```python
from build123d import *

# Parameters (mm, degrees)
SKETCH1_R           = 15
BOSS_EXTRUDE1_DEPTH = 35
SKETCH3_W           = 8
SKETCH3_H           = 45
CUT_EXTRUDE1_DEPTH  = 115
SKETCH5_R           = 30
BOSS_EXTRUDE2_DEPTH = 75


with BuildPart() as part:
    # Sketch1 → Boss-Extrude1 (new body)
    with BuildSketch(Plane.XY):
        with BuildLine():
            Line((-40, 107.819293264), (-40, -107.819293264))
            ThreePointArc((-40, -107.819293264), (0, -115), (40, -107.819293264))
            Line((40, -107.819293264), (40, 107.819293264))
            ThreePointArc((40, 107.819293264), (0, 115), (-40, 107.819293264))
        make_face()
        with Locations((0, 75)):
            Circle(SKETCH1_R, mode=Mode.SUBTRACT)
        with Locations((0, -75)):
            Circle(SKETCH1_R, mode=Mode.SUBTRACT)
    extrude(amount=BOSS_EXTRUDE1_DEPTH)

    # Sketch3 → Cut-Extrude1 (cut)
    with BuildSketch(Plane(origin=(40, 0, 0), x_dir=(0, 0, -1), z_dir=(1, 0, 0))):
        with Locations((-4, 0)):
            Rectangle(SKETCH3_W, SKETCH3_H)
    extrude(amount=-CUT_EXTRUDE1_DEPTH, mode=Mode.SUBTRACT)

    # Sketch5 → Boss-Extrude2 (add)
    with BuildSketch(Plane.XY.offset(35)):
        Circle(SKETCH5_R)
    extrude(amount=BOSS_EXTRUDE2_DEPTH)


solid = part.part
```
Can you work these out from the model? Positions are in its coordinate system, mm. A direction names the side the tool comes from. Give positions to 0.01 mm unless a question says otherwise; leave off trailing zeros. Loops run counter-clockwise (first coordinate to the right, second up) from the corner with the lowest first, then second, coordinate; pieces in that order, holes last. Notation, with made-up numbers: M 37,-31.75 L 93,-31.75 A5 cw 93,-23.75 Z; hole C 46,-33.5 d4. An arc over 180 degrees is marked long. Use one line per item in the form item = value. Start each with the question number.
(1) On a 3-axis mill with a long thin cutter (end or side, diameter ignored), from which of +Z, -Z, +X, -X, +Y, -Y can I reach the whole of each face in a straight line? I mean faces 4 (the cylindrical face through (-29.97, 1.32, 71.97)), 5 (the flat face through (1, -22.5, 4)), 6 (the flat face through (40, -2, 17)). Say none if no direction works.
(2) I want a section at B-B, the plane x = 0. Write out the boundary of the cut face in (y, z).
(3) I want a section at C-C, the plane z = 22.5. Write out the boundary of the cut face in (x, y), and give its area (3 significant figures).
(4) I'm going to push flat-ended pins straight in: P1, Ø5, axis at x = -4.5, z = 64, coming from the +Y side; P2, Ø12, axis at x = 21, z = 96, coming from the -Y side; P3, Ø3, axis at x = 7, z = 90, coming from the -Y side. Where does each tip first touch, or does it pass through?
(5) Please list where these lines run through material, in increasing order: line 1 (Y direction, x = 0, z = 13.5); line 2 (Z direction, x = 19, y = 78.5); line 3 (Z direction, x = 7.5, y = -12).
(6) Thinking about a two-plate mould opening in Y: for faces 1 (the cylindrical face through (-0.6, -115, 17.3)), 2 (the flat face through (1, 22.5, 4)), 3 (the cylindrical face through (0.6, 115, 17.3)), which applies, released by +Y, released by -Y, zero draft, split by the parting line, or undercut?
(7) I want a section at A-A, the plane y = 75. Write out the boundary of the cut face in (x, z).
(8) I want a section at D-D, the plane y = 0. Write out the boundary of the cut face in (x, z).
Worked out:
q1.face_4 = +Z
q1.face_5 = -Z, +X, -X
q1.face_6 = +Z, -Z, +X, +Y, -Y
q2.outline = M -115,0 L -90,0 L -90,35 L -115,35 Z; M -60,0 L -22.5,0 L -22.5,8 L 22.5,8 L 22.5,0 L 60,0 L 60,35 L 30,35 L 30,110 L -30,110 L -30,35 L -60,35 Z; M 90,0 L 115,0 L 115,35 L 90,35 Z
q3.outline = M -40,-107.82 A115 ccw 40,-107.82 L 40,107.82 A115 ccw -40,107.82 Z; hole C 0,-75 d30; hole C 0,75 d30
q3.area = 16,600 mm²
q4.P1 = 29.93
q4.P2 = -25.98
q4.P3 = -29.49
q5.line_1 = -115 to -90, -60 to 60, 90 to 115
q5.line_2 = 0 to 35
q5.line_3 = 8 to 110
q6.face_1 = released by -Y
q6.face_2 = undercut
q6.face_3 = released by +Y
q7.outline = M -40,0 L -15,0 L -15,35 L -40,35 Z; M 15,0 L 40,0 L 40,35 L 15,35 Z
q8.outline = M -40,8 L 40,8 L 40,35 L 30,35 L 30,110 L -30,110 L -30,35 L -40,35 Z
